from build123d import *

# Parameters (mm, degrees)
BOSS_EXTRUDE2_DEPTH   = 20
BOSS_EXTRUDE2_2_DEPTH = 20
SKETCH3_W             = 60
SKETCH3_H             = 50
BOSS_EXTRUDE3_DEPTH   = 3
SKETCH4_R             = 1.6
CUT_EXTRUDE1_DEPTH    = 10


with BuildPart() as part:
    # Sketch1 → Boss-Extrude2 (new body)
    with BuildSketch(Plane(origin=(0, 0, 0), x_dir=(1, 0, 0), z_dir=(0, 1, 0))):
        Polygon((-20.35, 22.2), (22.35, 22.2), (22.35, 24.2), (-22.35, 24.2), (-22.35, -4.7), (-29.7, -4.7), (-29.7, -9.4), (-27.7, -9.4), (-27.7, -6.7), (-20.35, -6.7), align=None)
    extrude(amount=BOSS_EXTRUDE2_DEPTH)



with BuildPart() as body_2:
    # Sketch1 → Boss-Extrude2 2 (new body)
    with BuildSketch(Plane(origin=(0, 0, 0), x_dir=(1, 0, 0), z_dir=(0, 1, 0))):
        Polygon((20.35, -6.7), (20.35, 10), (22.35, 10), (22.35, -4.7), (29.7, -4.7), (29.7, -9.4), (27.7, -9.4), (27.7, -6.7), align=None)
    extrude(amount=BOSS_EXTRUDE2_2_DEPTH)


with BuildPart() as part_1:
    add(part.part)

    add(body_2.part)  # Boss-Extrude3 merges body 2
    # Sketch3 → Boss-Extrude3 (add)
    with BuildSketch(Plane(origin=(0, 0, 0), x_dir=(1, 0, 0), z_dir=(0, 1, 0))):
        Rectangle(SKETCH3_W, SKETCH3_H)
    extrude(amount=-BOSS_EXTRUDE3_DEPTH)

    # Sketch4 → Cut-Extrude1 (cut)
    with BuildSketch(Plane.XY):
        with Locations((-24.3, 14.95)):
            Circle(SKETCH4_R)
        with Locations((24.3, 14.95)):
            Circle(SKETCH4_R)
        with Locations((24.3, 5.05)):
            Circle(SKETCH4_R)
        with Locations((-24.3, 5.05)):
            Circle(SKETCH4_R)
    extrude(amount=CUT_EXTRUDE1_DEPTH, mode=Mode.SUBTRACT)


solid = part_1.part
CAD build for the part. Positions are in the model's coordinates, mm. A direction names the side the tool comes from. Give positions to 0.01 mm unless a question says otherwise; leave off trailing zeros. Order: outer loops, then holes, each group sorted by start corner. A loop starts at its lowest first (then second) coordinate and runs counter-clockwise, first axis right, second up. Notation, with made-up numbers: (62.25, 21.5) -> (86.25, 21.5) arc R16 ccw to (86.25, 50.5) -> close; hole circle Ø10 at (83, -1.75). An arc over 180 degrees is marked (long way). Return JSON: item names as keys, results as strings.
Q1. Mould opens along X. For faces 1 (the face through (24, 10, 6.7)), 2 (the face through (22.35, 10, -23)), 3 (the face through (-9.6, 20, -22.4)) say: pulls with the +X half, pulls with the -X half, needs draft (parallel to the pull), parting line crosses it, or undercut.
Working result:
{"face 1": "undercut", "face 2": "pulls with the +X half", "face 3": "needs draft"}
Q2. Saw through at B-B (x = -24.3). Write the cut outline in (y, z).
Working result:
{"outline": "(-3, -25) -> (0, -25) -> (0, 4.7) -> (3.45, 4.7) -> (3.45, 6.7) -> (0, 6.7) -> (0, 25) -> (-3, 25) -> close; (6.65, 4.7) -> (13.35, 4.7) -> (13.35, 6.7) -> (6.65, 6.7) -> close; (16.55, 4.7) -> (20, 4.7) -> (20, 6.7) -> (16.55, 6.7) -> close"}
Q3. Saw through at A-A (y = 14.95). Write the cut outline in (x, z).
Working result:
{"outline": "(-29.7, 4.7) -> (-25.9, 4.7) -> (-25.9, 6.7) -> (-27.7, 6.7) -> (-27.7, 9.4) -> (-29.7, 9.4) -> close; (-22.7, 4.7) -> (-22.35, 4.7) -> (-22.35, -24.2) -> (22.35, -24.2) -> (22.35, -22.2) -> (-20.35, -22.2) -> (-20.35, 6.7) -> (-22.7, 6.7) -> close; (20.35, -10) -> (22.35, -10) -> (22.35, 4.7) -> (22.7, 4.7) -> (22.7, 6.7) -> (20.35, 6.7) -> close; (25.9, 4.7) -> (29.7, 4.7) -> (29.7, 9.4) -> (27.7, 9.4) -> (27.7, 6.7) -> (25.9, 6.7) -> close"}
Q4. Drill centre lines: line 1 (X direction, y = 5.05, z = 6.2); line 2 (Y direction, x = -24.3, z = 6.1); line 3 (X direction, y = 11.5, z = -8.5). Where is each one in solid material? Low to high.
Working result:
{"line 1": "-29.7 to -25.9, -22.7 to -20.35, 20.35 to 22.7, 25.9 to 29.7", "line 2": "-3 to 3.45, 6.65 to 13.35, 16.55 to 20", "line 3": "-22.35 to -20.35, 20.35 to 22.35"}
Q5. Saw through at C-C (y = 1.5). Write the cut outline in (x, z), then the cut area to 3 significant figures.
Working result:
{"outline": "(-29.7, 4.7) -> (-22.35, 4.7) -> (-22.35, -24.2) -> (22.35, -24.2) -> (22.35, -22.2) -> (-20.35, -22.2) -> (-20.35, 6.7) -> (-27.7, 6.7) -> (-27.7, 9.4) -> (-29.7, 9.4) -> close; (20.35, -10) -> (22.35, -10) -> (22.35, 4.7) -> (29.7, 4.7) -> (29.7, 9.4) -> (27.7, 9.4) -> (27.7, 6.7) -> (20.35, 6.7) -> close", "area": "221 mm²"}
Q6. Flat gauge pins, fed straight in: pin 1 (8 mm diameter, centred on y = 3, z = 2.5, fed in from +X); pin 2 (8 mm diameter, centred on y = 8, z = -15.5, fed in from +X); pin 3 (10 mm diameter, centred on y = 9, z = -7, fed in from -X); pin 4 (2 mm diameter, centred on x = -27, y = 11, fed in from -Z). Where does each tip first touch, or does it go through?
Working result:
{"pin 1": "x = 30", "pin 2": "x = -20.35", "pin 3": "x = -22.35", "pin 4": "z = 4.7"}
Q7. Which spindle directions (+Z, -Z, +X, -X, +Y, -Y) get a long thin tool onto all of the face, cutting with end or side? Do faces 4 (the face through (-20.35, 10, -8)), 5 (the face through (-29, 10, 9.4)), 6 (the face through (29.7, 10, 7)), 7 (the face through (21, 10, -10)). Say none if no direction does.
Working result:
{"face 4": "+Z, +Y", "face 5": "+Z, +X, -X, +Y", "face 6": "+Z, -Z, +X, +Y", "face 7": "+X, +Y"}
Q8. Saw through at D-D (z = -14). Write the cut outline in (x, y), then the cut area to 3 significant figures.
Working result:
{"outline": "(-30, -3) -> (30, -3) -> (30, 0) -> (-20.35, 0) -> (-20.35, 20) -> (-22.35, 20) -> (-22.35, 0) -> (-30, 0) -> close", "area": "220 mm²"}
